from build123d import *

# Parameters (mm, degrees)
SKETCH1_W           = 286.9
SKETCH1_H           = 21.5
SKETCH1_R           = 3
BOSS_EXTRUDE1_DEPTH = 4
SKETCH2_W           = 286.9
SKETCH2_H           = 12
BOSS_EXTRUDE2_DEPTH = 4
SKETCH6_R           = 1.55
CUT_EXTRUDE4_DEPTH  = 271.248330559


with BuildPart() as part:
    # Sketch1 → Boss-Extrude1 (new body)
    with BuildSketch(Plane(origin=(0, 0, 0), x_dir=(1, 0, 0), z_dir=(0, 1, 0))):
        with Locations((126.1, -6.4)):
            Rectangle(SKETCH1_W, SKETCH1_H)
        with Locations(Location((0, 0, 0), (0, 0, 270))):
            Circle(SKETCH1_R, mode=Mode.SUBTRACT)
        with Locations(Location((21.7, 0, 0), (0, 0, 270))):
            Circle(SKETCH1_R, mode=Mode.SUBTRACT)
        with Locations(Location((43.4, 0, 0), (0, 0, 270))):
            Circle(SKETCH1_R, mode=Mode.SUBTRACT)
        with Locations(Location((65.1, 0, 0), (0, 0, 270))):
            Circle(SKETCH1_R, mode=Mode.SUBTRACT)
        with Locations(Location((86.8, 0, 0), (0, 0, 270))):
            Circle(SKETCH1_R, mode=Mode.SUBTRACT)
        with Locations(Location((108.5, 0, 0), (0, 0, 270))):
            Circle(SKETCH1_R, mode=Mode.SUBTRACT)
        with Locations(Location((130.2, 0, 0), (0, 0, 270))):
            Circle(SKETCH1_R, mode=Mode.SUBTRACT)
        with Locations(Location((151.9, 0, 0), (0, 0, 270))):
            Circle(SKETCH1_R, mode=Mode.SUBTRACT)
        with Locations(Location((173.6, 0, 0), (0, 0, 270))):
            Circle(SKETCH1_R, mode=Mode.SUBTRACT)
        with Locations(Location((195.3, 0, 0), (0, 0, 270))):
            Circle(SKETCH1_R, mode=Mode.SUBTRACT)
        with Locations(Location((217, 0, 0), (0, 0, 270))):
            Circle(SKETCH1_R, mode=Mode.SUBTRACT)
        with Locations(Location((238.7, 0, 0), (0, 0, 270))):
            Circle(SKETCH1_R, mode=Mode.SUBTRACT)
    extrude(amount=BOSS_EXTRUDE1_DEPTH)

    # Sketch2 → Boss-Extrude2 (add)
    with BuildSketch(Plane.XY.offset(17.15)):
        with Locations((126.1, 10)):
            Rectangle(SKETCH2_W, SKETCH2_H)
    extrude(amount=-BOSS_EXTRUDE2_DEPTH)

    # Sketch6 → Cut-Extrude4 (cut, through all)
    with BuildSketch(Plane(origin=(0, 8.408785298, 13.15), x_dir=(-1, 0, 0), z_dir=(0, 0, 1))):
        with Locations(Location((-262.05, 0.408785298, 0), (0, 0, 180))):
            Circle(SKETCH6_R)
        with Locations(Location((-248.55, 0.408785298, 0), (0, 0, 180))):
            Circle(SKETCH6_R)
        with Locations(Location((9.85, 0.408785298, 0), (0, 0, 180))):
            Circle(SKETCH6_R)
    extrude(amount=CUT_EXTRUDE4_DEPTH, mode=Mode.SUBTRACT)


solid = part.part
The model under review builds one solid part; all positions refer to its coordinate system, in mm. A direction names the side the tool comes from. Round coordinates to 2 decimals unless told otherwise and drop trailing zeros. Loops run counter-clockwise (first coordinate to the right, second up) from the corner with the lowest first, then second, coordinate; pieces in that order, holes last. Notation, with made-up numbers: (58, -13) -> (68, -13) arc R18 cw to (68, -2) -> close; hole circle Ø5 at (68, -15). An arc over 180 degrees is marked (long way). Return JSON: item names as keys, results as strings.
(1) For pin 1 (5.5 mm diameter, centred on x = 65.1, z = 0, fed in from -Y); pin 2 (9.5 mm diameter, centred on x = 217, z = 0, fed in from +Y); pin 3 (1 mm diameter, centred on x = 111.5, z = 0, fed in from -Y), all flat-tipped, find the tip position at first contact; note any pin that passes through.
Solved:
{"pin 1": "through", "pin 2": "y = 4", "pin 3": "y = 0"}
(2) Add section A-A on x = 151.9. Write out the cut boundary in (y, z), plus the area to 3 significant figures.
Solved:
{"outline": "(0, -4.35) -> (4, -4.35) -> (4, -3) -> (0, -3) -> close; (0, 3) -> (4, 3) -> (4, 13.15) -> (16, 13.15) -> (16, 17.15) -> (0, 17.15) -> close", "area": "110 mm2"}
(3) For faces 1 (the flat face through (124, 10, 13.15)), 2 (the cylindrical face through (0.9, 1.97, 2.86)), list the 3-axis set-ups (+Z, -Z, +X, -X, +Y, -Y) from which the entire face can be reached by the end or side of a thin tool; tool diameter is ignored.
Solved:
{"face 1": "-Z, +X, -X, +Y", "face 2": "+Y, -Y"}
(4) Add section B-B on x = 5.5. Write out the cut boundary in (y, z).
Solved:
{"outline": "(0, -4.35) -> (4, -4.35) -> (4, 13.15) -> (16, 13.15) -> (16, 17.15) -> (0, 17.15) -> close"}
(5) For line 1 (X direction, y = 8, z = 14.75); line 2 (Y direction, x = -9.85, z = 16.05); line 3 (Y direction, x = 119.5, z = 6.25), list the stretches that pass through material, from the lowest coordinate up.
Solved:
{"line 1": "-17.35 to -11.4, -8.3 to 247, 250.1 to 260.5, 263.6 to 269.55", "line 2": "0 to 6.45, 9.55 to 16", "line 3": "0 to 4"}
(6) The part is to be moulded in two halves that separate along Z. For faces 3 (the flat face through (124, 8, 17.15)), 4 (the flat face through (124, 0, 6)), 5 (the cylindrical face through (132.73, 1.97, 1.61)), say which applies: released by +Z, released by -Z, zero draft, split by the parting line, or undercut.
Solved:
{"face 3": "released by +Z", "face 4": "zero draft", "face 5": "undercut"}
(7) Add section C-C on z = 9. Write out the cut boundary in (x, y), plus the area to 3 significant figures.
Solved:
{"outline": "(-17.35, 0) -> (269.55, 0) -> (269.55, 4) -> (-17.35, 4) -> close", "area": "1,150 mm2"}
